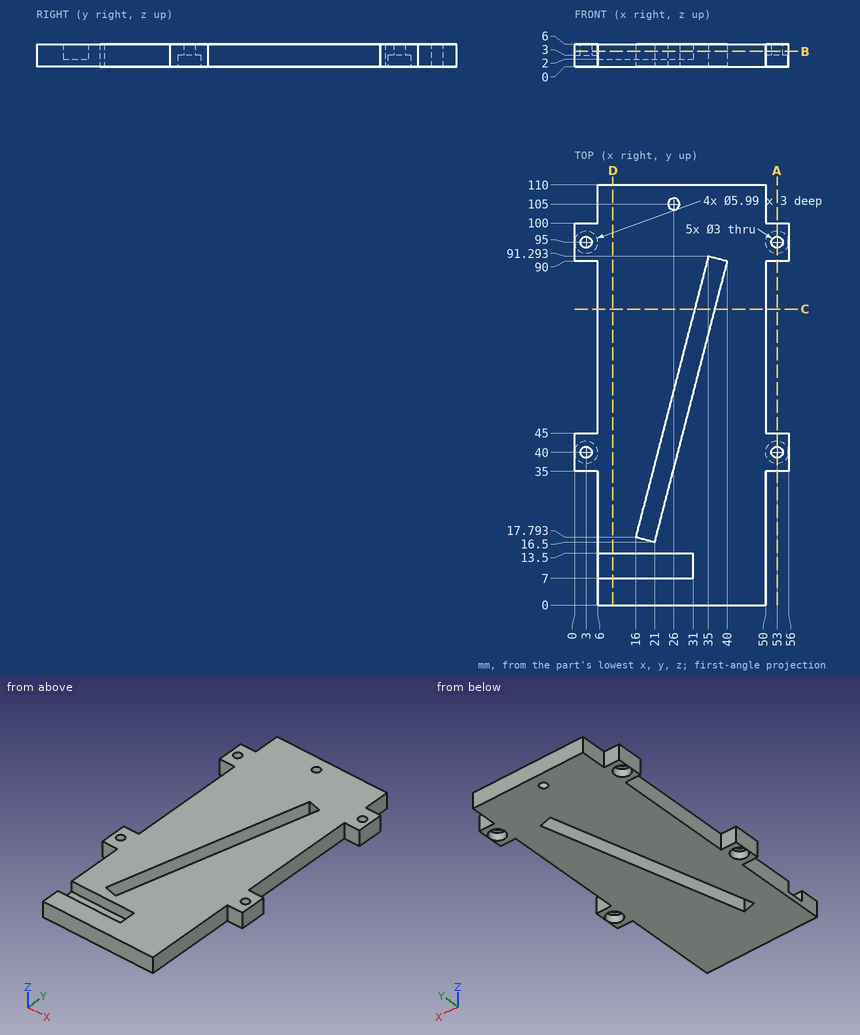
The drawing under review shows one solid part. Ordinate dimensions are in mm from its lowest x, y, z. Coordinates: 2 decimals unless noted, no trailing zeros. Write each loop counter-clockwise with the first axis right and the second up, starting at its lowest first coordinate (ties: lowest second). Pieces come first, ordered by that corner, then holes.
1) Add section D-D (x = 10). Write out the cut boundary in (y, z), plus the area to 3 significant figures.
2) Add section B-B (z = 4.05). State how many separate pieces and enclosed holes the cut face has, plus the area to 3 significant figures.
3) Add section C-C (y = 77.5). Write out the cut boundary in (x, z) (1 decimal).
4) To check wall thickness, follow L1, parallel to Y at x = 3, z = 4.45; L2, parallel to Y at x = 53, z = 2.15 (1 decimal); L3, parallel to X at y = 95, z = 4.5. State the ranges of each line that lie inside material, in increasing order.
5) Add section A-A (x = 53). Write out the cut boundary in (y, z) (1 decimal).
6) Insertion check: pin 1 (1.8 mm diameter, centred on x = 3.5, z = 2, fed in from +Y); pin 2 (4 mm diameter, centred on x = 23.5, y = 45.5, fed in from +Z); pin 3 (5 mm diameter, centred on x = 3, y = 40, fed in from -Z); pin 4 (3 mm diameter, centred on y = 20.5, z = 2, fed in from -X). Each pin has a flat end and moves straight along its axis. Give the tip position at first contact, or say it passes through.
Check result:
1. outline: (0, 0) - (110, 0) - (110, 6) - (13.5, 6) - (13.5, 2) - (7, 2) - (7, 6) - (0, 6) - close
1. area: 634 mm2
2. separate pieces: 1
2. enclosed holes: 6
2. area: 4,490 mm2
3. outline: (6, 0) - (31.4, 0) - (31.4, 6) - (6, 6) - close; (36.8, 0) - (50, 0) - (50, 6) - (36.8, 6) - close
4. L1: y = 35 to 38.5, 41.5 to 45, 90 to 93.5, 96.5 to 100
4. L2: y = 35 to 37, 43 to 45, 90 to 92, 98 to 100
4. L3: x = 0 to 1.5, 4.5 to 51.5, 54.5 to 56
5. outline: (35, 0) - (37, 0) - (37, 3) - (38.5, 3) - (38.5, 6) - (35, 6) - close; (41.5, 3) - (43, 3) - (43, 0) - (45, 0) - (45, 6) - (41.5, 6) - close; (90, 0) - (92, 0) - (92, 3) - (93.5, 3) - (93.5, 6) - (90, 6) - close; (96.5, 3) - (98, 3) - (98, 0) - (100, 0) - (100, 6) - (96.5, 6) - close
6. pin 1: stops at y = 100
6. pin 2: stops at z = 6
6. pin 3: stops at z = 3
6. pin 4: stops at x = 6
